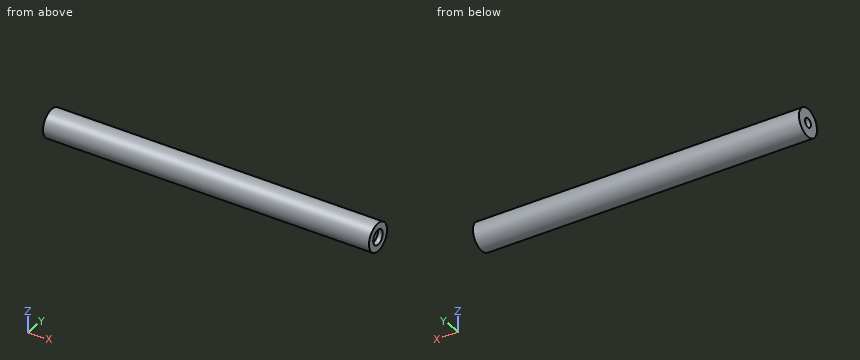
from build123d import *

# Parameters (mm, degrees)
SKETCH1_R           = 8.636
BOSS_EXTRUDE1_DEPTH = 203.2
SKETCH2_R           = 4.572
CUT_EXTRUDE1_DEPTH  = 3.048
SKETCH3_R           = 2.794
CUT_EXTRUDE2_DEPTH  = 14.478


with BuildPart() as part:
    # Sketch1 → Boss-Extrude1 (new body)
    with BuildSketch(Plane(origin=(0, 0, 0), x_dir=(0, 0, -1), z_dir=(1, 0, 0))):
        Circle(SKETCH1_R)
    extrude(amount=BOSS_EXTRUDE1_DEPTH)

    # Sketch2 → Cut-Extrude1 (cut)
    with BuildSketch(Plane(origin=(203.2, 0, 0), x_dir=(0, 0, -1), z_dir=(1, 0, 0))):
        Circle(SKETCH2_R)
    extrude(amount=-CUT_EXTRUDE1_DEPTH, mode=Mode.SUBTRACT)

    # Sketch3 → Cut-Extrude2 (cut)
    with BuildSketch(Plane.ZY):
        Circle(SKETCH3_R)
    extrude(amount=-CUT_EXTRUDE2_DEPTH, mode=Mode.SUBTRACT)


solid = part.part
Check sheet for the modelled part. Datum: model origin and axes. Units: mm. Give positions to 0.01 mm unless a question says otherwise; leave off trailing zeros. Write each loop counter-clockwise with the first axis right and the second up, starting at its lowest first coordinate (ties: lowest second). Pieces come first, ordered by that corner, then holes. Notation, with made-up numbers: (-1, -24.5) -> (12, -24.5) arc R25 cw to (12, -7.5) -> close; hole circle Ø10 at (64, 59). An arc over 180 degrees is marked (long way). One line per item, written item: value. Start each with the question number.
Item 1: Section check C-C on x = 52. Record the cut outline in (y, z), then the cut area to 3 significant figures.
Item 2: Section check A-A on z = 0. Record the cut outline in (x, y).
Item 3: Material ranges on probe 1 along Y at (x, z) = (7.75, 0); probe 2 along Y at (x, z) = (202.3, 0); probe 3 along Z at (x, y) = (155, -0.5), recorded low to high. Write a range as from..to.
Item 4: Gauge pin test, flat ends, axial feed: pin 1 (3 mm diameter, centred on x = 63, z = 3, fed in from -Y); pin 2 (1.7 mm diameter, centred on y = 1, z = -0.5, fed in from -X); pin 3 (10 mm diameter, centred on x = 182, y = -5.5, fed in from -Z). Record the tip position at first contact, or that the pin passes through.
Results list:
1. outline: circle Ø17.27 at (0, 0)
1. area: 234 mm²
2. outline: (0, -8.64) -> (203.2, -8.64) -> (203.2, -4.57) -> (200.15, -4.57) -> (200.15, 4.57) -> (203.2, 4.57) -> (203.2, 8.64) -> (0, 8.64) -> (0, 2.79) -> (14.48, 2.79) -> (14.48, -2.79) -> (0, -2.79) -> close
3. probe 1: -8.64..-2.79, 2.79..8.64
3. probe 2: -8.64..-4.57, 4.57..8.64
3. probe 3: -8.62..8.62
4. pin 1: y = -8.5
4. pin 2: x = 14.48
4. pin 3: z = -8.62
